Source: CAD feature listing. Evaluate the final solid. Frame: model axes, mm. A direction names the side the tool comes from. Give positions to 0.01 mm unless a question says otherwise; leave off trailing zeros. Order: outer loops, then holes, each group sorted by start corner. A loop starts at its lowest first (then second) coordinate and runs counter-clockwise, first axis right, second up.
1) Section C-C, the plane z = 6. Return loops of the section in (x, y), plus the area to 3 significant figures.
2) Section B-B, the plane z = 28. Return loops of the section in (x, y).
3) Draft query along Y for faces 1 (the face through (23.289, 14.804, 19.72)), 2 (the face through (64.381, -32.915, 4.93)), 3 (the face through (87.064, -48.73, 4.93)), 4 (the face through (24.78, -39.57, 4.93)). Return one class per face: released by +Y, released by -Y, zero draft, split by the parting line, or undercut.
4) Access query for faces 5 (the face through (11, 0, 25)), 6 (the face through (79, 13, 20)), 7 (the face through (54, -34, 10)), 8 (the face through (56, -3, 25)), 9 (the face through (0, -4, 6)). Directions: +Z, -Z, +X, -X, +Y, -Y. A direction counts if a zero-diameter tool reaches every point of the face in a straight line with its end or side. Return the directions, or none.
5) First-contact query: P1, Ø11, axis at x = 8.5, z = 20.5, coming from the -Y side; P2, Ø5.5, axis at x = 5.5, z = 25, coming from the +Y side; P3, Ø11, axis at x = 30.5, z = 29, coming from the -Y side. Flat tips, straight axial feed; report the tip coordinate or a pass-through.
6) Material intervals for line 1 (X direction, y = -31, z = 3); line 2 (Y direction, x = 76, z = 19.5); line 3 (X direction, y = 19, z = 20.5), sorted ascending.
7) Section D-D, the plane x = 7. Return loops of the section in (y, z).
Autodesk Fusion 360 part; units mm, degrees
sketch "Sketch" plane through (0, 0, 0) normal (0, 0, 1) x (-1, 0, 0)
  line L0 (-88, 67) -> (0, 67)
  line L1 (0, 67) -> (0, 0)
  line L2 (0, 0) -> (-88, 0)
  line L3 (-88, 0) -> (-88, 67)
  circle A0 centre (-19, 31) radius 5
  circle A1 centre (-69, 31) radius 5
  line L4 (-44, 67) -> (-30.7145, 80.5829) construction
  arc A2 (-30.7145, 80.5829) -> (-57.5829, 80.2855) centre (-44, 67) ccw
  line L5 (-44, 67) -> (-57.5829, 80.2855) construction
  line L6 (-44, 67) -> (-30.7145, 80.5829) construction
  line L7 (-30.7145, 80.5829) -> (0, 50.5408)
  line L8 (-57.5829, 80.2855) -> (-88, 49.1876)
  circle A3 centre (-13, 45.0716) radius 13
  circle A4 centre (-75, 43.8869) radius 13
  line L9 (0, 0) -> (-88, 0)
  line L10 (-63, 3) -> (-25, 3)
  circle A5 centre (-22, 3) radius 3
  circle A6 centre (-66, 3) radius 3
  line L11 (-25, 3) -> (-63, 3)
  line L12 (0, -13) -> (0, 0)
  line L13 (-88, -13) -> (0, -13)
  line L14 (0, 0) -> (-88, 0)
  line L15 (-88, 0) -> (-88, -13)
  line L16 (-44, 67) -> (-39, 67)
  line L17 (-39, 67) -> (-49, 67)
  line L18 (-39, 3) -> (-39, 67)
  line L19 (-49, 67) -> (-49, 3)
  line L20 (-49, 3) -> (-39, 3)
  line L21 (-49, 3) -> (-49, 7)
  line L22 (-39, 3) -> (-49, 3)
  line L23 (-39, 7) -> (-39, 3)
  line L24 (-49, 7) -> (-39, 7)
  circle A7 centre (-44, -19) radius 9.5
  circle A8 centre (-44, -19) radius 19
  line L25 (-44, -13) -> (-44, -19)
  line L26 (0, -13) -> (-44, -13)
  circle A9 centre (-19, -19) radius 6
  line L27 (-44, -13) -> (-44, -19)
  line L28 (-88, -13) -> (-44, -13)
  circle A10 centre (-69, -19) radius 6
  point P0 (-70.5776, 67)
  point P1 (-16.8276, 67)
  dimension "d1" = 67
  dimension "d6" = 10
  dimension "d7" = 10
  dimension "d11" = 19
  dimension "d12" = 50
  dimension "d13" = 13
  dimension "d14" = 13
  dimension "d15" = 88
  dimension "d25" = 31
  dimension "d30" = 3
  dimension "d31" = 3
  dimension "d32" = 38
  dimension "d33" = 13
  dimension "d35" = 64
  dimension "d36" = 10
  dimension "d37" = 4
  dimension "d39" = 19
  dimension "d40" = 19
  dimension "d41" = 38
  dimension "d42" = 6
  dimension "d43" = 6
extrude "Extrude2" add sketch "Sketch" along normal blind 10 contours L0 A2 L7 L8 L16 L17 | L0 L2 L3 A1 L8 A4 L9 L10 A6 L11 L14 L19 L21 | L0 L1 L2 A0 L7 A3 L9 L10 A5 L11 L14 L18 L23 | A1 A4 | A6 | A5 | A0 A3 picked at (-77.2796, 48.9706) picked at (-18.9905, 30.8691)
extrude "Extrude3" add sketch "Sketch" along normal blind 40 contours L0 L16 L17 L18 L19 L24
chamfer "Chamfer1" distance 60 distance2 30 1 edges at (44, -67, 40) measured on face at (45.6667, -47, 40)
extrude "Extrude4" add sketch "Sketch" along normal blind 40 contours L10 L11 L18 L19 L20 L21 L22 L23 L24 | L2 L9 L10 A5 A6 L11 L14 L20 L22 | L2 L9 L13 L14 L15 A8 L28 | L2 L9 L12 L13 L14 A8 L26 | L13 A7 A8 L26 L28 | L13 A8 L28 A10 | L13 A7 A8 L26 L28 | L13 A8 L26 A9
extrude "Extrude5" cut sketch "Sketch" along normal blind 50 contours A10
From the geometry:
1. outline: (0, -45.07) arc R13 cw (long way) to (3.93, -54.39) - (30.71, -80.58) arc R19 ccw to (57.58, -80.29) - (84.29, -52.98) arc R13 ccw to (88, -43.89) - (88, 13) - (69, 13) arc R6 cw to (63, 19) arc R19 ccw to (25, 19) arc R6 cw to (19, 13) - (0, 13) - close; hole circle Ø19 at (44, 19); hole circle Ø10 at (69, -31)
1. area: 7,300 mm2
2. outline: (0, 0) - (22, 0) arc R3 cw to (25, -3) - (39, -3) - (39, -31.01) - (49, -31.01) - (49, -3) - (63, -3) arc R3 cw to (66, 0) - (88, 0) - (88, 13) - (69, 13) arc R6 cw to (63, 19) arc R19 ccw to (25, 19) arc R6 cw to (19, 13) - (0, 13) - close; hole circle Ø19 at (44, 19)
3. face 1: released by +Y
3. face 2: undercut
3. face 3: released by -Y
3. face 4: undercut
4. face 5: +Z, -X, -Y
4. face 6: +Z, -Z, +X, +Y
4. face 7: +Z, -Y
4. face 8: +Z, +X, -Y
4. face 9: +Z, -Z, -X, +Y, -Y
5. P1: stops at y = 0
5. P2: stops at y = 13
5. P3: stops at y = -3
6. line 1: x = 0 to 64, 74 to 88
6. line 2: y = 0 to 13
6. line 3: x = 25 to 34.5, 53.5 to 63
7. outline: (-57.39, 0) - (-56.6, 0) - (-56.6, 10) - (-57.39, 10) - close; (-33.54, 0) - (13, 0) - (13, 40) - (0, 40) - (0, 10) - (-33.54, 10) - close
